from build123d import *

# Parameters (mm, degrees)
CROQUIS2_W              = 90
CROQUIS2_H              = 55
CROQUIS2_W_2            = 80
CROQUIS2_H_2            = 45
SALIENTE_EXTRUIR2_DEPTH = 12.5
CROQUIS4_R              = 3.5
CORTAR_EXTRUIR2_DEPTH   = 86
CROQUIS5_R              = 2
CROQUIS5_R_2            = 2.5
CORTAR_EXTRUIR4_DEPTH   = 10


with BuildPart() as part:
    # Croquis2 → Saliente-Extruir2 (new body, symmetric)
    with BuildSketch(Plane.XY):
        with Locations((45, 27.5)):
            Rectangle(CROQUIS2_W, CROQUIS2_H)
        with Locations((45, 27.5)):
            Rectangle(CROQUIS2_W_2, CROQUIS2_H_2, mode=Mode.SUBTRACT)
    extrude(amount=SALIENTE_EXTRUIR2_DEPTH, both=True)

    # Croquis4 → Cortar-Extruir2 (cut)
    with BuildSketch(Plane(origin=(90, 0, 0), x_dir=(0, 0, -1), z_dir=(1, 0, 0))):
        with Locations((0, 18.5)):
            Circle(CROQUIS4_R)
    extrude(amount=-CORTAR_EXTRUIR2_DEPTH, mode=Mode.SUBTRACT)

    # Croquis5 → Cortar-Extruir4 (cut)
    with BuildSketch(Plane(origin=(0, 55, 0), x_dir=(1, 0, 0), z_dir=(0, 1, 0))):
        with Locations((20, 0)):
            Circle(CROQUIS5_R)
        with Locations((62, 0)):
            Circle(CROQUIS5_R_2)
    extrude(amount=-CORTAR_EXTRUIR4_DEPTH, mode=Mode.SUBTRACT)


solid = part.part
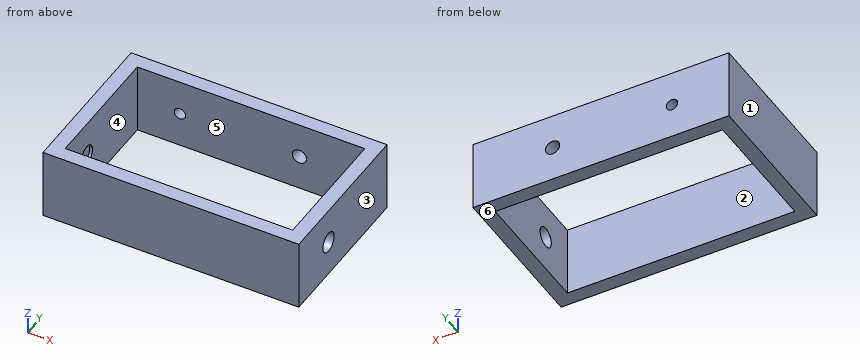
Could you check a few things on this model? Use its own coordinates, in mm. Face numbers are marked on the shaded views. A direction names the side the tool comes from. Round coordinates to 2 decimals unless told otherwise and drop trailing zeros. Order: outer loops, then holes, each group sorted by start corner. A loop starts at its lowest first (then second) coordinate and runs counter-clockwise, first axis right, second up.
(1) Please list where these lines run through material, in increasing order: line 1 along X through (y, z) = (44, -7.75); line 2 along Y through (x, z) = (16, 6.25); line 3 along Y through (x, z) = (4.6, 0).
Response values:
line 1: x = 0 to 5, 85 to 90
line 2: y = 0 to 5, 50 to 55
line 3: y = 0 to 15, 22 to 55
(2) If we mould it in two halves opening along X, with no side actions, what happens to the marked faces 1, 2, 3 and 4? For each: released by +X, released by -X, zero draft, split by the parting line, or undercut.
Response values:
face 1: released by -X
face 2: undercut
face 3: released by +X
face 4: undercut
(3) Which directions (+Z, -Z, +X, -X, +Y, -Y) give clear straight access to the entire face, cutting with the end or side of a thin tool? Please do the marked faces 5 and 6.
Response values:
face 5: +Z, -Z
face 6: -Z, +X, -X, +Y, -Y
(4) Imagine slicing it at A-A (x = 56.5). Write out the boundary of the cut face in (y, z).
Response values:
outline: (0, -12.5) - (5, -12.5) - (5, 12.5) - (0, 12.5) - close; (50, -12.5) - (55, -12.5) - (55, 12.5) - (50, 12.5) - close
(5) Imagine slicing it at B-B (z = 0). Write out the boundary of the cut face in (x, y), plus the area to 3 significant figures.
Response values:
outline: (0, 0) - (90, 0) - (90, 15) - (85, 15) - (85, 5) - (5, 5) - (5, 15) - (4, 15) - (4, 22) - (5, 22) - (5, 50) - (18, 50) - (18, 55) - (0, 55) - close; (22, 50) - (59.5, 50) - (59.5, 55) - (22, 55) - close; (64.5, 50) - (85, 50) - (85, 22) - (90, 22) - (90, 55) - (64.5, 55) - close
area: 1,260 mm2
(6) Imagine slicing it at C-C (x = 20). Write out the boundary of the cut face in (y, z).
Response values:
outline: (0, -12.5) - (5, -12.5) - (5, 12.5) - (0, 12.5) - close; (50, -12.5) - (55, -12.5) - (55, -2) - (50, -2) - close; (50, 2) - (55, 2) - (55, 12.5) - (50, 12.5) - close
(7) Imagine slicing it at D-D (y = 18.5). Write out the boundary of the cut face in (x, z).
Response values:
outline: (0, -12.5) - (5, -12.5) - (5, -3.5) - (4, -3.5) - (4, 3.5) - (5, 3.5) - (5, 12.5) - (0, 12.5) - close; (85, -12.5) - (90, -12.5) - (90, -3.5) - (85, -3.5) - close; (85, 3.5) - (90, 3.5) - (90, 12.5) - (85, 12.5) - close
